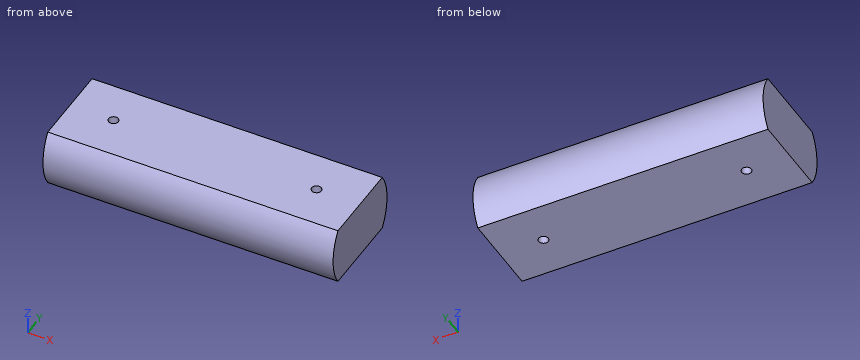
Autodesk Inventor part; units mm, degrees
ref_plane "YZ Plane" through (0, 0, 0) normal (1, 0, 0) x (0, 1, 0)
ref_plane "XZ Plane" through (0, 0, 0) normal (0, 1, 0) x (-1, 0, 0)
ref_plane "XY Plane" through (0, 0, 0) normal (0, 0, 1) x (1, 0, 0)
sketch "Sketch1" plane through (0, 0, 0) normal (0, 0, 1) x (1, 0, 0)
  line L0 (0, 0) -> (100, 0)
  line L1 (100, 0) -> (100, 17.5)
  line L2 (100, 17.5) -> (0, 17.5)
  line L3 (0, 17.5) -> (0, 0)
  dimension "d0" = 100
  dimension "d1" = 17.5
revolve "Revolution1" add sketch "Sketch1" angle 360 about axis through (0, 0, 0) along (1, 0, 0)
sketch "Sketch2" plane through (100, 0, 0) normal (1, 0, 0) x (0, 0, -1)
  line L0 (-22.6333, 22.279) -> (-10, 22.279)
  line L1 (-10, 22.279) -> (-10, -22.279)
  line L2 (-10, -22.279) -> (-22.6333, -22.279)
  line L3 (-22.6333, -22.279) -> (-22.6333, 22.279)
  line L4 (10, 22.279) -> (22.1679, 22.279)
  line L5 (22.1679, 22.279) -> (22.1679, -28.0835)
  line L6 (22.1679, -28.0835) -> (10, -28.0835)
  line L7 (10, -28.0835) -> (10, 22.279)
  circle A0 centre (0, 0) radius 17.5
  dimension "d3" = 50.3625
  dimension "d4" = 44.558
  dimension "d5" = 20
  dimension "d6" = 10
  dimension "d7" = 22.279
  dimension "d8" = 12.1679
  dimension "d9" = 12.6333
  dimension "d22" = 35
extrude "Extrusion1" cut sketch "Sketch2" against normal through all contours L0 L1 A0 L2 L3 | L1 A0 | A0 L7 | L7 L4 L5 L6 A0
sketch "Sketch3" plane through (100, -14.3614, 10) normal (0, 0, 1) x (1, 0, 0)
  line L0 (0, 28.7228) -> (0, 0)
  line L1 (-100, 0) -> (-100, 28.7228)
  point P0 (-100, 14.3614)
  point P1 (-85, 14.3614)
  point P2 (-15, 14.3614)
  point P3 (0, 14.3614)
  dimension "d12" = 15
  dimension "d13" = 15
  dimension "d14" = 70
hole "Hole1" at (15, 0, 10) at (85, 0, 10) direction (0, 0, -1) diameter 3.302 end through all
properties part number "Top_Lever Handle" material "Wood (Oak)"
Source: CAD feature listing. Evaluate the final solid. Frame: model axes, mm. Give positions to 0.01 mm unless a question says otherwise; leave off trailing zeros. Loops run counter-clockwise (first coordinate to the right, second up) from the corner with the lowest first, then second, coordinate; pieces in that order, holes last. Notation, with made-up numbers: (19.25, 46) -> (48.25, 46) arc R30 ccw to (48.25, 70) -> close; hole circle Ø8 at (23.5, 11). An arc over 180 degrees is marked (long way). Use a Markdown table: item, result. Add a question column.
(1) Section query A-A (y = 0). Output: boundary loops of the cut face in (x, z).
(2) Section query B-B (x = 85). Output: boundary loops of the cut face in (y, z).
(3) Section query C-C (z = -8). Output: boundary loops of the cut face in (x, y).
(4) First-contact query: pin 1 Ø4 at (x, z) = (29.5, -2) entering from +Y. Flat tip, straight axial feed; report the tip coordinate or a pass-through.
(5) Ray query, line 1 (X direction, y = 0, z = 5); line 2 (Y direction, x = 78, z = 0.5); line 3 (Y direction, x = 15, z = 2.25). Return the intervals inside material, ascending.
Checked values:
| question | item | result |
|---|---|---|
| 1 | outline | (0, -10) -> (13.35, -10) -> (13.35, 10) -> (0, 10) -> close; (16.65, -10) -> (83.35, -10) -> (83.35, 10) -> (16.65, 10) -> close; (86.65, -10) -> (100, -10) -> (100, 10) -> (86.65, 10) -> close |
| 2 | outline | (-14.36, -10) -> (-1.65, -10) -> (-1.65, 10) -> (-14.36, 10) arc R17.5 ccw to start; (1.65, -10) -> (14.36, -10) arc R17.5 ccw to (14.36, 10) -> (1.65, 10) -> close |
| 3 | outline | (0, -15.56) -> (100, -15.56) -> (100, 15.56) -> (0, 15.56) -> close; hole circle Ø3.3 at (15, 0); hole circle Ø3.3 at (85, 0) |
| 4 | pin 1 | y = 17.5 |
| 5 | line 1 | 0 to 13.35, 16.65 to 83.35, 86.65 to 100 |
| 5 | line 2 | -17.49 to 17.49 |
| 5 | line 3 | -17.35 to -1.65, 1.65 to 17.35 |
